from build123d import *

# Parameters (mm, degrees)
F1_DEPTH = 20
F2_W     = 40
F2_H     = 20
F3_DEPTH = 40
F5_DEPTH = 40
F6_W     = 20
F6_H     = 30
F7_DEPTH = 25


with BuildPart() as f1:
    # F0 (on Right) → F1 (new body)
    with BuildSketch(Plane.YZ):
        Polygon((-3.7623762107, 0), (36.2376237893, 0), (36.2376237893, 40), (16.2376237893, 40), (-3.7623762107, 20), align=None)
    extrude(amount=-F1_DEPTH)

    # F2 (on face) → F3 (join)
    with BuildSketch(Plane(origin=(-20, 0, 0), x_dir=(0, -1, 0), z_dir=(-1, 0, 0))):
        with Locations((-16.2376237893, 10)):
            Rectangle(F2_W, F2_H)
    extrude(amount=F3_DEPTH)

    # F4 (on face) → F5 (cut)
    with BuildSketch(Plane(origin=(-60, 0, 0), x_dir=(0, -1, 0), z_dir=(-1, 0, 0))):
        Polygon((3.7623762107, 20), (-16.2376237893, 20), (3.7623762107, 0), align=None)
    extrude(amount=-F5_DEPTH, mode=Mode.SUBTRACT)

    # F6 (on face) → F7 (cut)
    with BuildSketch(Plane(origin=(0, 0, 0), x_dir=(1, 0, 0), z_dir=(0, 0, -1))):
        with Locations((-30, -11.2376237893)):
            Rectangle(F6_W, F6_H)
    extrude(amount=-F7_DEPTH, mode=Mode.SUBTRACT)


solid = f1.part
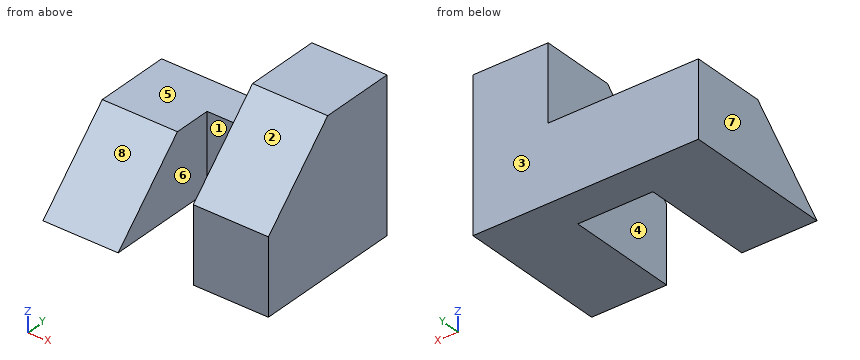
CAD build for the part. Positions are in the model's coordinates, mm. Face numbers are marked on the shaded views. A direction names the side the tool comes from. Round coordinates to 2 decimals unless told otherwise and drop trailing zeros. Order: outer loops, then holes, each group sorted by start corner. A loop starts at its lowest first (then second) coordinate and runs counter-clockwise, first axis right, second up. Notation, with made-up numbers: (60, -40) - (70, -40) arc R9 cw to (70, -33) - close; hole circle Ø6 at (-9, 0.25). An arc over 180 degrees is marked (long way). Return JSON: item names as keys, results as strings.
(1) Pin check, flat tips, straight feed: pin 1 Ø3 at (y, z) = (29.5, 29) entering from +X; pin 2 Ø12 at (x, z) = (-32, 24.5) entering from -Y; pin 3 Ø2 at (x, y) = (-53, 19.5) entering from +Z; pin 4 Ø2 at (y, z) = (32, 33) entering from -X. Stop position of each tip, or through.
Answer key:
{"pin 1": "stops at x = 0", "pin 2": "stops at y = 26.24", "pin 3": "stops at z = 20", "pin 4": "stops at x = -20"}
(2) Cut at D-D (y = 14). Give the cut face in (x, z).
Answer key:
{"outline": "(-60, 0) - (-40, 0) - (-40, 17.76) - (-60, 17.76) - close; (-20, 0) - (0, 0) - (0, 37.76) - (-20, 37.76) - close"}
(3) Cut at C-C (x = -14.5). Give the cut face in (y, z).
Answer key:
{"outline": "(-3.76, 0) - (36.24, 0) - (36.24, 40) - (16.24, 40) - (-3.76, 20) - close"}
(4) Cut at A-A (y = 23.5). Give the cut face in (x, z), then the cut area to 3 significant figures.
Answer key:
{"outline": "(-60, 0) - (-40, 0) - (-40, 20) - (-60, 20) - close; (-20, 0) - (0, 0) - (0, 40) - (-20, 40) - close", "area": "1,200 mm^2"}
(5) Tool access for the marked faces 1, 2, 3, 4 and 5: list every direction of +Z, -Z, +X, -X, +Y, -Y with a clear straight run to the whole face (end or side of a thin tool).
Answer key:
{"face 1": "+Z, -Z, -Y", "face 2": "+Z, +X, -X, -Y", "face 3": "+Z, -Z, +X, -X, +Y", "face 4": "+Z, -Y", "face 5": "+Z, -X, +Y, -Y"}
(6) Pull direction X, two halves, no side cores. Call the marked faces 6, 7 and 8: +X half, -X half, draft (parallel to the pull), parting line (faces both ways), or undercut.
Answer key:
{"face 6": "undercut", "face 7": "-X half", "face 8": "draft"}
(7) Cut at B-B (z = 14.5). Give the cut face in (x, y).
Answer key:
{"outline": "(-60, 10.74) - (-40, 10.74) - (-40, 26.24) - (-20, 26.24) - (-20, -3.76) - (0, -3.76) - (0, 36.24) - (-60, 36.24) - close"}
(8) Wall check: probe 1 along X at (y, z) = (17.5, 15); probe 2 along Y at (x, z) = (-26, 12.5); probe 3 along Z at (x, y) = (-33, 32). Give the ranges that are in metal, low to high. Write a range as from..to.
Answer key:
{"probe 1": "x = -60..-40, -20..0", "probe 2": "y = 26.24..36.24", "probe 3": "z = 0..20"}
